Geometry: final body of the model. Coordinates: model frame, mm. A direction names the side the tool comes from. Round coordinates to 2 decimals unless told otherwise and drop trailing zeros. Loops run counter-clockwise (first coordinate to the right, second up) from the corner with the lowest first, then second, coordinate; pieces in that order, holes last. Notation, with made-up numbers: M -28,-2 L -18,-2 A28 ccw -18,24 Z; hole C 56.5,10.5 d9. An arc over 180 degrees is marked long. Answer as a JSON object with one key per item and string values.
from build123d import *

# Parameters (mm, degrees)
SKETCH002_R     = 8.1
PAD001_DEPTH    = 5
SKETCH_W        = 15
SKETCH_H        = 30
PAD_DEPTH       = 12.1
SKETCH001_R     = 6.2
POCKET_DEPTH    = 15.001
SKETCH003_R     = 1.5
POCKET001_DEPTH = 12.101
POCKET002_DEPTH = 2.5
SKETCH005_W     = 30
SKETCH005_H     = 12.1
PAD002_DEPTH    = 2.5
SKETCH006_R     = 8.2
POCKET003_DEPTH = 2.5
SKETCH007_W     = 15
SKETCH007_H     = 12.1
PAD003_DEPTH    = 8
SKETCH008_W     = 15
SKETCH008_H     = 12.1
PAD004_DEPTH    = 8
SKETCH009_R     = 1.5
POCKET004_DEPTH = 12.101
POCKET005_DEPTH = 2.5


with BuildPart() as pad001:
    # Sketch002 → Pad001 (new body, symmetric)
    with BuildSketch(Plane.YZ):
        with Locations((0, 12)):
            Circle(SKETCH002_R)
    extrude(amount=PAD001_DEPTH, both=True)


with BuildPart() as pocket005:
    # Sketch → Pad (new body)
    with BuildSketch(Plane.XY):
        Rectangle(SKETCH_W, SKETCH_H)
    extrude(amount=PAD_DEPTH)

    # Sketch001 → Pocket (cut, through all)
    with BuildSketch(Plane.YZ.offset(7.5)):
        with Locations((0, 12)):
            Circle(SKETCH001_R)
    extrude(amount=-POCKET_DEPTH, mode=Mode.SUBTRACT)

    # Cut: cut Pad001
    add(pad001.part, mode=Mode.SUBTRACT)

    # Sketch003 → Pocket001 (cut, through all)
    with BuildSketch(Plane(origin=(0, 0, 0), x_dir=(1, 0, 0), z_dir=(0, 0, -1))):
        with Locations((0, 11.5)):
            Circle(SKETCH003_R)
        with Locations((0, -11.5)):
            Circle(SKETCH003_R)
    extrude(amount=-POCKET001_DEPTH, mode=Mode.SUBTRACT)

    # Sketch004 → Pocket002 (cut)
    with BuildSketch(Plane(origin=(0, 0, 0), x_dir=(1, 0, 0), z_dir=(0, 0, -1))):
        Polygon((3.2, 11.5), (1.6, 14.271281), (-1.6, 14.271281), (-3.2, 11.5), (-1.6, 8.728719), (1.6, 8.728719), align=None)
        Polygon((1.6, -14.271281), (3.2, -11.5), (1.6, -8.728719), (-1.6, -8.728719), (-3.2, -11.5), (-1.6, -14.271281), align=None)
    extrude(amount=-POCKET002_DEPTH, mode=Mode.SUBTRACT)

    # Sketch005 → Pad002 (new body)
    with BuildSketch(Plane(origin=(-7.5, 0, 0), x_dir=(0, -1, 0), z_dir=(-1, 0, 0))):
        with Locations((0, 6.05)):
            Rectangle(SKETCH005_W, SKETCH005_H)
    extrude(amount=PAD002_DEPTH)

    # Sketch006 → Pocket003 (cut)
    with BuildSketch(Plane(origin=(-10, 0, 0), x_dir=(0, -1, 0), z_dir=(-1, 0, 0))):
        with Locations((0, 12.016602)):
            Circle(SKETCH006_R)
    extrude(amount=-POCKET003_DEPTH, mode=Mode.SUBTRACT)

    # Sketch007 → Pad003 (new body)
    with BuildSketch(Plane.XZ.offset(15)):
        with Locations((0, 6.05)):
            Rectangle(SKETCH007_W, SKETCH007_H)
    extrude(amount=PAD003_DEPTH)

    # Sketch008 → Pad004 (new body)
    with BuildSketch(Plane(origin=(0, 15, 0), x_dir=(-1, 0, 0), z_dir=(0, 1, 0))):
        with Locations((0, 6.05)):
            Rectangle(SKETCH008_W, SKETCH008_H)
    extrude(amount=PAD004_DEPTH)

    # Sketch009 → Pocket004 (cut, through all)
    with BuildSketch(Plane.XY.offset(12.1)):
        with Locations((0, -19)):
            Circle(SKETCH009_R)
        with Locations((0, 19)):
            Circle(SKETCH009_R)
    extrude(amount=-POCKET004_DEPTH, mode=Mode.SUBTRACT)

    # Sketch010 → Pocket005 (cut)
    with BuildSketch(Plane.XY.offset(12.1)):
        Polygon((1.6, -21.771281), (3.2, -19), (1.6, -16.228719), (-1.6, -16.228719), (-3.2, -19), (-1.6, -21.771281), align=None)
        Polygon((1.6, 16.228719), (3.2, 19), (1.6, 21.771281), (-1.6, 21.771281), (-3.2, 19), (-1.6, 16.228719), align=None)
    extrude(amount=-POCKET005_DEPTH, mode=Mode.SUBTRACT)


solid = pocket005.part
1) Reachability of faces 5 (the flat face through (-9, -15, 6)), 6 (the flat face through (-7.5, -0.6, 5.5)), 7 (the flat face through (-2.389, -12.905, 1.232)), 8 (the flat face through (-5, 0, 5.6)) from +Z, -Z, +X, -X, +Y, -Y: full face, straight path, thin tool, end or side. Return the list, or none.
Results:
{"face 5": "+Z, -Z, -X, -Y", "face 6": "+Z, -X", "face 7": "-Z", "face 8": "+Z"}
2) Section query D-D (x = 0). Count the separate pieces of the cut face and the enclosed holes in it, and give its area (3 significant figures).
Results:
{"separate pieces": "5", "enclosed holes": "0", "area": "281 mm2"}
3) Pin query (flat end, axial travel): P1, Ø4, axis at x = 0, y = 4, coming from the +Z side; P2, Ø2.5, axis at y = 21, z = 7.5, coming from the -X side; P3, Ø5, axis at x = 0, y = -11.5, coming from the -Z side; P4, Ø1.8, axis at x = 0, y = 19, coming from the +Z side. Return the tip coordinate at first contact, or that it passes through.
Results:
{"P1": "z = 6.56", "P2": "x = -7.5", "P3": "z = 2.5", "P4": "through"}
4) Section query B-B (y = 0). Return the cut outline in (x, z).
Results:
{"outline": "M -10,0 L 7.5,0 L 7.5,5.8 L 5,5.8 L 5,3.9 L -5,3.9 L -5,5.8 L -7.5,5.8 L -7.5,3.82 L -10,3.82 Z"}
5) Section query A-A (z = 6.75). Return the cut outline in (x, y).
Results:
{"outline": "M -10,-15 L -7.5,-15 L -7.5,-23 L 7.5,-23 L 7.5,-3.3 L 5,-3.3 L 5,-6.17 L -5,-6.17 L -5,-3.3 L -7.5,-3.3 L -7.5,-6.29 L -10,-6.29 Z; M -10,6.29 L -7.5,6.29 L -7.5,3.3 L -5,3.3 L -5,6.17 L 5,6.17 L 5,3.3 L 7.5,3.3 L 7.5,23 L -7.5,23 L -7.5,15 L -10,15 Z; hole C 0,-19 d3; hole C 0,-11.5 d3; hole C 0,11.5 d3; hole C 0,19 d3"}
6) Ray query, line 1 (X direction, y = -7, z = 9.75); line 2 (X direction, y = -11.5, z = 4.75); line 3 (Y direction, x = 0, z = 5). Return the intervals inside material, ascending.
Results:
{"line 1": "-7.5 to -5, 5 to 7.5", "line 2": "-10 to -1.5, 1.5 to 7.5", "line 3": "-23 to -20.5, -17.5 to -13, -10 to -4.08, 4.08 to 10, 13 to 17.5, 20.5 to 23"}
7) Pull-direction query (Y, two-part tool) for faces 1 (the cylindrical face through (0.07, -0.18, 3.9)), 2 (the flat face through (-7.5, 19, 6)), 3 (the flat face through (2.389, -20.405, 10.868)), 4 (the flat face through (0, -23, 6)); classes: +Y half, -Y half, draft (parallel to the pull), parting line (faces both ways), or undercut.
Results:
{"face 1": "undercut", "face 2": "draft", "face 3": "undercut", "face 4": "-Y half"}
8) Section query C-C (z = 3). Return the cut outline in (x, y).
Results:
{"outline": "M -10,-15 L -7.5,-15 L -7.5,-23 L 7.5,-23 L 7.5,23 L -7.5,23 L -7.5,15 L -10,15 Z; hole C 0,-19 d3; hole C 0,-11.5 d3; hole C 0,11.5 d3; hole C 0,19 d3"}
